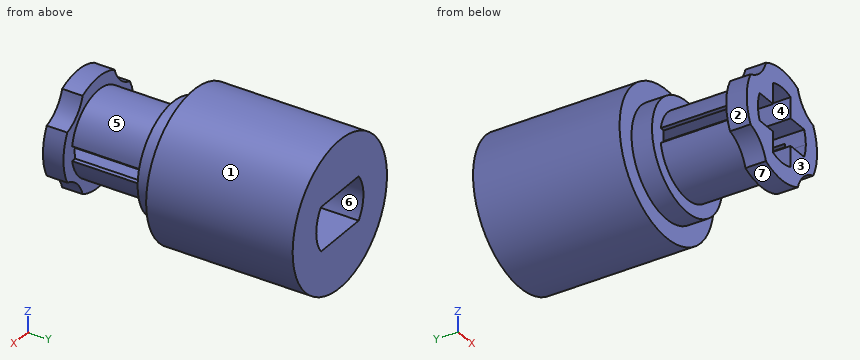
from build123d import *

# Parameters (mm, degrees)
F0_R      = 3.73
F3_DEPTH  = 1.4
F2_R      = 2.85
F4_DEPTH  = 1.4
F1_R      = 2.85
F5_DEPTH  = 7.86
F6_DEPTH  = 7.86
F7_DEPTH  = 7.86
F8_DEPTH  = 7.86
F9_DEPTH  = 7.86
F10_R     = 2.85
F11_DEPTH = 1.4
F12_W     = 5.06
F12_H     = 1
F13_DEPTH = 8
F14_W     = 5.06
F14_H     = 1
F15_DEPTH = 8
F17_R     = 5
F18_DEPTH = 10
F20_DEPTH = 6.5


with BuildPart() as f3:
    # F0 (on Front) → F3 (new body)
    with BuildSketch(Plane.XZ):
        Circle(F0_R)
    extrude(amount=F3_DEPTH)

    # F2 (on Front) → F4 (cut)
    with BuildSketch(Plane.XZ):
        Circle(F2_R)
    extrude(amount=F4_DEPTH, mode=Mode.SUBTRACT)

    # F1 (on Front) → F5 (join)
    with BuildSketch(Plane.XZ):
        Circle(F1_R)
        with BuildLine():
            ThreePointArc((-0.93, 2.36), (0, 2.536632), (0.93, 2.36))
            ThreePointArc((0.93, 2.36), (1.793669, 1.793669), (2.36, 0.93))
            ThreePointArc((2.36, 0.93), (2.492083, 0.473312), (2.536632, 0))
            ThreePointArc((2.536632, 0), (2.492083, -0.473312), (2.36, -0.93))
            ThreePointArc((2.36, -0.93), (1.793669, -1.793669), (0.93, -2.36))
            ThreePointArc((0.93, -2.36), (0, -2.536632), (-0.93, -2.36))
            ThreePointArc((-0.93, -2.36), (-1.793669, -1.793669), (-2.36, -0.93))
            ThreePointArc((-2.36, -0.93), (-2.536632, 0), (-2.36, 0.93))
            ThreePointArc((-2.36, 0.93), (-1.793669, 1.793669), (-0.93, 2.36))
        make_face(mode=Mode.SUBTRACT)
    extrude(amount=F5_DEPTH)

    # F1 (on Front) → F6 (join)
    with BuildSketch(Plane.XZ):
        with BuildLine():
            ThreePointArc((2.36, 0.93), (1.793669, 1.793669), (0.93, 2.36))
            Line((0.93, 2.36), (0.93, 0.93))
            Line((0.93, 0.93), (2.36, 0.93))
        make_face()
    extrude(amount=F6_DEPTH)

    # F1 (on Front) → F7 (join)
    with BuildSketch(Plane.XZ):
        with BuildLine():
            Line((-0.93, -0.93), (-2.36, -0.93))
            ThreePointArc((-2.36, -0.93), (-1.793669, -1.793669), (-0.93, -2.36))
            Line((-0.93, -2.36), (-0.93, -0.93))
        make_face()
    extrude(amount=F7_DEPTH)

    # F1 (on Front) → F8 (join)
    with BuildSketch(Plane.XZ):
        with BuildLine():
            Line((-0.93, 0.93), (-0.93, 2.36))
            ThreePointArc((-0.93, 2.36), (-1.793669, 1.793669), (-2.36, 0.93))
            Line((-2.36, 0.93), (-0.93, 0.93))
        make_face()
    extrude(amount=F8_DEPTH)

    # F1 (on Front) → F9 (join)
    with BuildSketch(Plane.XZ):
        with BuildLine():
            ThreePointArc((0.93, -2.36), (1.793669, -1.793669), (2.36, -0.93))
            Line((2.36, -0.93), (0.93, -0.93))
            Line((0.93, -0.93), (0.93, -2.36))
        make_face()
    extrude(amount=F9_DEPTH)

    # F10 (on face) → F11 (join)
    with BuildSketch(Plane.XZ.offset(7.86)):
        with BuildLine():
            ThreePointArc((-1.691716, 3.324304), (-2.301731, 2.301731), (-3.324304, 1.691716))
            ThreePointArc((-3.324304, 1.691716), (-3.73, 0), (-3.324304, -1.691716))
            ThreePointArc((-3.324304, -1.691716), (-2.301731, -2.301731), (-1.691716, -3.324304))
            ThreePointArc((-1.691716, -3.324304), (0, -3.73), (1.691716, -3.324304))
            ThreePointArc((1.691716, -3.324304), (2.301731, -2.301731), (3.324304, -1.691716))
            ThreePointArc((3.324304, -1.691716), (3.73, 0), (3.324304, 1.691716))
            ThreePointArc((3.324304, 1.691716), (2.301731, 2.301731), (1.691716, 3.324304))
            ThreePointArc((1.691716, 3.324304), (0, 3.73), (-1.691716, 3.324304))
        make_face()
        Circle(F10_R, mode=Mode.SUBTRACT)
    extrude(amount=-F11_DEPTH)

    # F12 (on Right) → F13 (cut)
    with BuildSketch(Plane.YZ):
        with Locations((-3.93, 0)):
            Rectangle(F12_W, F12_H)
    extrude(amount=-F13_DEPTH, mode=Mode.SUBTRACT)

    # F14 (on Right) → F15 (cut)
    with BuildSketch(Plane.YZ):
        with Locations((-3.93, 0)):
            Rectangle(F14_W, F14_H)
    extrude(amount=F15_DEPTH, mode=Mode.SUBTRACT)

    # F17 (on offset) → F18 (join)
    with BuildSketch(Plane.XZ.offset(-10)):
        Circle(F17_R)
    extrude(amount=F18_DEPTH)

    # F19 (on offset) → F20 (cut)
    with BuildSketch(Plane.XZ.offset(-10)):
        with BuildLine():
            Line((2, 1.5), (-2, 1.5))
            ThreePointArc((-2, 1.5), (-2.5, 0), (-2, -1.5))
            Line((-2, -1.5), (2, -1.5))
            ThreePointArc((2, -1.5), (2.5, 0), (2, 1.5))
        make_face()
    extrude(amount=F20_DEPTH, mode=Mode.SUBTRACT)


solid = f3.part
The listing builds one solid part. Answer for the finished solid, in the listing's coordinates (mm). Face numbers are marked on the shaded views. A direction names the side the tool comes from. Coordinates: 2 decimals unless noted, no trailing zeros. Order: outer loops, then holes, each group sorted by start corner. A loop starts at its lowest first (then second) coordinate and runs counter-clockwise, first axis right, second up. Notation, with made-up numbers: (7, -25) -> (23, -25) arc R13 cw to (23, -14) -> close; hole circle Ø2 at (-13.5, 11). An arc over 180 degrees is marked (long way). Answer in a Markdown table with one row per item. Add a question column.
Item 1: Each of these flat-tipped pins is pushed along its axis until it touches: P1, Ø0.7, axis at y = -3.5, z = 1.5, coming from the +X side; P2, Ø0.7, axis at x = 1.5, y = -2, coming from the +Z side; P3, Ø1.6, axis at x = 1.5, y = -6, coming from the -Z side; P4, Ø3.5, axis at x = -0.5, z = -0.5, coming from the +Y side. Where does it stop, or does it pass through?
Item 2: Find section B-B (x = 0). Write down the section's boundary in (y, z), then the cut area to 3 significant figures.
Item 3: Find section C-C (y = 8). Write down the section's boundary in (x, z), then the cut area to 3 significant figures.
Item 4: Find section A-A (y = -2.5). Write down the section's boundary in (x, z).
Item 5: Find section D-D (z = -0.25). Write down the section's boundary in (x, y), then the cut area to 3 significant figures.
Item 6: Determine the mould class of the marked faces 1, 2, 3 and 4 for opening direction X: +X half, -X half, draft (parallel to the pull), parting line (faces both ways), or undercut.
Item 7: Find the intervals of material crossed by L1, parallel to Z at x = 0.5, y = -3.25; L2, parallel to Z at x = -1.75, y = -6; L3, parallel to Y at x = -4.5, z = -0.25, in increasing order. Write a range as from..to.
Item 8: Which of the six approach directions +Z, -Z, +X, -X, +Y, -Y give full straight-line access (tool end or side, diameter ignored) to the marked faces 5, 6 and 7?
Result set:
| question | item | result |
|---|---|---|
| 1 | P1 | stops at x = 2.61 |
| 1 | P2 | stops at z = 2.61 |
| 1 | P3 | stops at z = -3.63 |
| 1 | P4 | stops at y = 10 |
| 2 | outline | (-7.86, -3.73) -> (-6.46, -3.73) -> (-6.46, -2.85) -> (-1.4, -2.85) -> (-1.4, -3.73) -> (0, -3.73) -> (0, -5) -> (10, -5) -> (10, -1.5) -> (3.5, -1.5) -> (3.5, 1.5) -> (10, 1.5) -> (10, 5) -> (0, 5) -> (0, 3.73) -> (-1.4, 3.73) -> (-1.4, 2.85) -> (-6.46, 2.85) -> (-6.46, 3.73) -> (-7.86, 3.73) -> (-7.86, 2.54) -> (0, 2.54) -> (0, -2.54) -> (-7.86, -2.54) -> close |
| 2 | area | 90.4 mm² |
| 3 | outline | circle Ø10 at (0, 0); hole (-2, -1.5) -> (2, -1.5) arc R2.5 ccw to (2, 1.5) -> (-2, 1.5) arc R2.5 ccw to start |
| 3 | area | 64.5 mm² |
| 4 | outline | (-2.81, -0.5) arc R2.85 ccw to (2.81, -0.5) -> (2.49, -0.5) arc R2.54 cw to (2.36, -0.93) -> (0.93, -0.93) -> (0.93, -2.36) arc R2.54 cw to (-0.93, -2.36) -> (-0.93, -0.93) -> (-2.36, -0.93) arc R2.54 cw to (-2.49, -0.5) -> close; (-2.81, 0.5) -> (-2.49, 0.5) arc R2.54 cw to (-2.36, 0.93) -> (-0.93, 0.93) -> (-0.93, 2.36) arc R2.54 cw to (0.93, 2.36) -> (0.93, 0.93) -> (2.36, 0.93) arc R2.54 cw to (2.49, 0.5) -> (2.81, 0.5) arc R2.85 ccw to start |
| 5 | outline | (-4.99, 0) -> (-3.72, 0) -> (-3.72, -1.4) -> (-2.52, -1.4) -> (-2.52, 0) -> (2.52, 0) -> (2.52, -1.4) -> (3.72, -1.4) -> (3.72, 0) -> (4.99, 0) -> (4.99, 10) -> (2.49, 10) -> (2.49, 3.5) -> (-2.49, 3.5) -> (-2.49, 10) -> (-4.99, 10) -> close; (-3.72, -7.86) -> (-2.52, -7.86) -> (-2.52, -6.46) -> (-3.72, -6.46) -> close; (2.52, -7.86) -> (3.72, -7.86) -> (3.72, -6.46) -> (2.52, -6.46) -> close |
| 5 | area | 74.2 mm² |
| 6 | face 1 | parting line |
| 6 | face 2 | -X half |
| 6 | face 3 | draft |
| 6 | face 4 | undercut |
| 7 | L1 | z = -2.81..-2.49, 2.49..2.81 |
| 7 | L2 | z = -2.25..-0.93, 0.93..2.25 |
| 7 | L3 | y = 0..10 |
| 8 | face 5 | +Z |
| 8 | face 6 | +Y |
| 8 | face 7 | -Z, -Y |
